```python
from build123d import *

# Parameters (mm, degrees)
F1_DEPTH      = 13
F2_W          = 13
F2_H          = 10.75
F3_DEPTH      = 38.501
F4_R          = 1.75
F5_DEPTH      = 11.501
F5_DEPTH_BACK = 11.501
F6_R          = 2.75
F7_DEPTH      = 2.65
F8_DEPTH      = 1.55
F8_DEPTH_BACK = 14.55
F9_SIZE2      = 0.294734
F9_SIZE       = 1.09999
F10_DEPTH     = 2.6
F12_DEPTH     = 10.751
F13_R         = 6
F14_R         = 1
F15_R         = 1.75
F16_DEPTH     = 2.251


# Not quite as in the source:
# - a fillet or chamfer is up to 0.001 mm smaller than in the source, because OpenCascade refuses the exact size
# - a pattern or mirror of a feature is missing from the dataset's text; its kind, count and spacing are read off the source's solid


with BuildPart() as f1:
    # F0 (on Top) → F1 (new body)
    with BuildSketch(Plane.XY):
        Polygon((6.5, 30), (0, 30), (-6.5, 30), (-6.5, 38.5), (-11.5, 38.5), (-11.5, -2.6), (-6.5, -2.6), (-6.5, 0), (0, 0), (6.5, 0), (6.5, -2.6), (11.5, -2.6), (11.5, 38.5), (6.5, 38.5), align=None)
    extrude(amount=F1_DEPTH)

    # F2 (on Front) → F3 (cut, through all)
    with BuildSketch(Plane.XZ):
        with Locations((0, 7.625)):
            Rectangle(F2_W, F2_H)
    extrude(amount=-F3_DEPTH, mode=Mode.SUBTRACT)

    # F4 (on Right) → F5 (cut, two sides)
    with BuildSketch(Plane.YZ) as f5_sk:
        with BuildLine():
            Line((38.5, 6.5), (38.5, 13))
            Line((38.5, 13), (33.5533008589, 13))
            Line((33.5533008589, 13), (37.4016504294, 9.1516504294))
            ThreePointArc((37.4016504294, 9.1516504294), (38.2145482469, 7.9350628714), (38.5, 6.5))
        make_face()
        with Locations((4.4, 6.5)):
            Circle(F4_R)
        with Locations((14.4, 6.5)):
            Circle(F4_R)
        with BuildLine():
            ThreePointArc((21.2931220671, 12.9516726658), (21.8460337805, 12.9879124141), (22.4, 13))
            Line((22.4, 13), (-2.6, 13))
            Line((-2.6, 13), (-2.6, 7.1959706526))
            ThreePointArc((-2.6, 7.1959706526), (-1.5491093472, 9.898331483), (1.051377029, 11.1807494449))
            Line((1.051377029, 11.1807494449), (21.2931220671, 12.9516726658))
        make_face()
    extrude(amount=-F5_DEPTH, mode=Mode.SUBTRACT)
    extrude(f5_sk.sketch, amount=F5_DEPTH_BACK, mode=Mode.SUBTRACT)

    # F6 (on face) → F7 (cut)
    with BuildSketch(Plane(origin=(6.5, 0, 0), x_dir=(0, -1, 0), z_dir=(-1, 0, 0))):
        with BuildLine():
            Line((-38.5, 0), (-30, 0))
            Line((-30, 0), (-30, 8.9638140898))
            Line((-30, 8.9638140898), (-29.2883115249, 13))
            Line((-29.2883115249, 13), (-33.5533008589, 13))
            Line((-33.5533008589, 13), (-37.4016504294, 9.1516504294))
            ThreePointArc((-37.4016504294, 9.1516504294), (-38.2145482469, 7.9350628714), (-38.5, 6.5))
            Line((-38.5, 6.5), (-38.5, 0))
        make_face()
        with Locations((-34.75, 6.5)):
            Circle(F6_R, mode=Mode.SUBTRACT)
    f7 = extrude(amount=-F7_DEPTH, mode=Mode.SUBTRACT)

    # F7_copies: F7 across plane
    add(f7.mirror(Plane(origin=(0, 0, 0), x_dir=(0, 0, -1), z_dir=(-1, 0, 0))), mode=Mode.SUBTRACT)

    # F8 (cut, two sides): a face of the model
    f8_faces = [f1.faces().sort_by_distance(p)[0] for p in [
        (6.5, 34.75, 6.5),
    ]]
    extrude(f8_faces, amount=-F8_DEPTH, mode=Mode.SUBTRACT)
    extrude(f8_faces, amount=F8_DEPTH_BACK, mode=Mode.SUBTRACT)

    # F9 (size 1.1 and 0.2947441117 in the source; OpenCascade refuses exactly that, so slightly less here)
    f9_edges = [f1.edges().sort_by_distance(p)[0] for p in [
        (8.05, 37.5, 6.5),
        (-8.05, 37.5, 6.5),
    ]]
    chamfer(f9_edges, length=F9_SIZE, length2=F9_SIZE2)

    # F10 (add, through all): a face of the model
    f10_faces = [f1.faces().sort_by_distance(p)[0] for p in [
        (0, 0, 1.125),
    ]]
    extrude(f10_faces, amount=F10_DEPTH)

    # F11 (on face) → F12 (cut, through all)
    with BuildSketch(Plane.XY.offset(2.25)):
        Polygon((-9.25, -2.6), (9.25, -2.6), (9.25, 20.3609127035), (6.5, 27), (-6.5, 27), (-9.25, 20.3609127035), align=None)
    extrude(amount=F12_DEPTH, mode=Mode.SUBTRACT)

    # F13
    f13_edges = [f1.edges().sort_by_distance(p)[0] for p in [
        (6.5, 27, 7.625),
        (9.25, 20.360913, 7.560057),
        (-6.5, 27, 7.625),
        (-9.25, 20.360913, 7.560057),
    ]]
    fillet(f13_edges, radius=F13_R)

    # F14
    f14_edges = [f1.edges().sort_by_distance(p)[0] for p in [
        (9.25, 8.283719, 2.25),
        (-9.25, 8.283719, 2.25),
        (6.5, 29.096737, 2.25),
        (6.615288, 27.022932, 2.25),
        (7.875, 23.680456, 2.25),
        (-6.5, 29.096737, 2.25),
        (9.134712, 20.33798, 2.25),
        (-6.615288, 27.022932, 2.25),
        (-7.875, 23.680456, 2.25),
        (-9.134712, 20.33798, 2.25),
    ]]
    fillet(f14_edges, radius=F14_R)

    # F15 (on face) → F16 (cut, through all)
    with BuildSketch(Plane.XY.offset(2.25)):
        with Locations((0, 4.4)):
            Circle(F15_R)
        with Locations((0, 14.4)):
            Circle(F15_R)
    extrude(amount=-F16_DEPTH, mode=Mode.SUBTRACT)


solid = f1.part
```
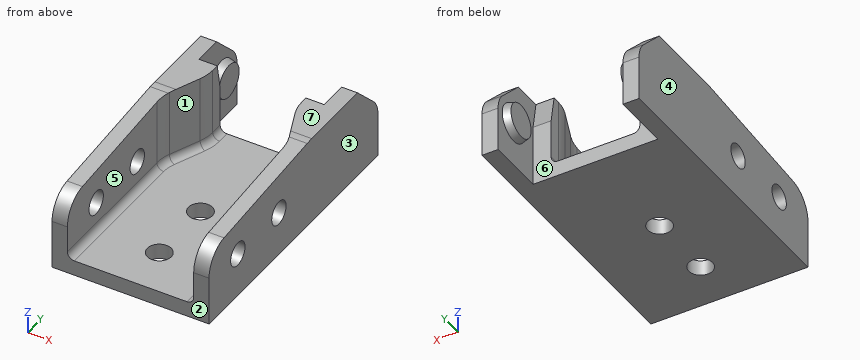
Geometry: final body of the model. Coordinates: model frame, mm. Face numbers are marked on the shaded views. A direction names the side the tool comes from. Round coordinates to 2 decimals unless told otherwise and drop trailing zeros. Order: outer loops, then holes, each group sorted by start corner. A loop starts at its lowest first (then second) coordinate and runs counter-clockwise, first axis right, second up. Notation, with made-up numbers: M -10.75,34 L 4.25,34 A18 ccw 4.25,38 Z; hole C 12,60.25 d6. An arc over 180 degrees is marked long. One line per item, written item: value.
(1) Cut plane A-A (x = 0). Return the cut outline in (y, z), and give its area (3 significant figures).
Result sheet:
outline: M -2.6,0 L 2.65,0 L 2.65,2.25 L -2.6,2.25 Z; M 6.15,0 L 12.65,0 L 12.65,2.25 L 6.15,2.25 Z; M 16.15,0 L 30,0 L 30,2.25 L 16.15,2.25 Z
area: 57.6 mm2
(2) Cut plane B-B (z = 11.75). Return the cut outline in (x, y).
Result sheet:
outline: M -11.5,7.56 L -9.25,7.56 L -9.25,19.17 A6 cw -8.79,21.46 L -6.96,25.9 A6 ccw -6.5,28.19 L -6.5,29.51 L -9.15,29.51 L -9.15,34.8 L -11.5,34.8 Z; M 6.5,28.19 A6 ccw 6.96,25.9 L 8.79,21.46 A6 cw 9.25,19.17 L 9.25,7.56 L 11.5,7.56 L 11.5,34.8 L 9.15,34.8 L 9.15,29.51 L 6.5,29.51 Z
(3) Pin query (flat end, axial travel): P1, Ø2, axis at x = 0, y = 4.4, coming from the -Z side; P2, Ø2, axis at x = -8.5, z = 10, coming from the -Y side; P3, Ø5, axis at x = -3, y = 18, coming from the +Z side; P4, Ø8, axis at x = -4.5, y = 10, coming from the +Z side. Return the tip coordinate at first contact, or that it passes through.
Result sheet:
P1: through
P2: y = -1.98
P3: z = 2.25
P4: z = 2.28
(4) Pull-direction query (X, two-part tool) for the marked faces 1, 2, 3 and 4; classes: pulls with the +X half, pulls with the -X half, needs draft (parallel to the pull), parting line crosses it, or undercut.
Result sheet:
face 1: undercut
face 2: needs draft
face 3: pulls with the +X half
face 4: pulls with the -X half
(5) Cut plane D-D (z = 1.5). Return the cut outline in (x, y).
Result sheet:
outline: M -11.5,-2.6 L 11.5,-2.6 L 11.5,38.5 L 9.15,38.5 L 9.15,30 L -9.15,30 L -9.15,38.5 L -11.5,38.5 Z; hole C 0,4.4 d3.5; hole C 0,14.4 d3.5
(6) Line query: probe 1 along Y at (x, z) = (10.2, 6.5); probe 2 along X at (y, z) = (7, 6.5); probe 3 along Y at (x, z) = (-10, 8). Output: solid intervals per line, ascending. Write a range as [from, to].
Result sheet:
probe 1: [-2.6, 2.65], [6.15, 12.65], [16.15, 38.5]
probe 2: [-11.5, -9.25], [9.25, 11.5]
probe 3: [-2.52, 3.5], [5.3, 13.5], [15.3, 38.19]
(7) Reachability of the marked faces 5, 6 and 7 from +Z, -Z, +X, -X, +Y, -Y: full face, straight path, thin tool, end or side. Return the list, or none.
Result sheet:
face 5: +Z, -Y
face 6: +Z, -Z
face 7: +Z, +X, -X, +Y, -Y
